Work out the finished part from the listing and answer in its coordinate system (mm). Round coordinates to 2 decimals unless told otherwise and drop trailing zeros. Loops run counter-clockwise (first coordinate to the right, second up) from the corner with the lowest first, then second, coordinate; pieces in that order, holes last. Notation, with made-up numbers: (61.25, 34.25) - (90.25, 34.25) arc R29 cw to (90.25, 57.25) - close; hole circle Ø9 at (-29, 7.25). An arc over 180 degrees is marked (long way). Return JSON: item names as keys, results as strings.
from build123d import *

# Parameters (mm, degrees)
EXTRUDE_1_DEPTH     = 3
SKETCH_2_R          = 1.5
CUT_EXTRUDE_1_DEPTH = 3
SKETCH_3_W          = 11
SKETCH_3_H          = 29.457142857
CUT_EXTRUDE_2_DEPTH = 3
SKETCH_4_W          = 11
SKETCH_4_H          = 29.457142857
CUT_EXTRUDE_3_DEPTH = 3
CUT_EXTRUDE_4_DEPTH = 3


with BuildPart() as part:
    # 草图1 → 凸台-拉伸1 (new body)
    with BuildSketch(Plane.XY):
        Polygon((0, 0), (15, 0), (32.5, -23), (32.5, -38), (-17.5, -38), (-17.5, -23), align=None)
    extrude(amount=EXTRUDE_1_DEPTH)

    # 草图2 → 切除-拉伸1 (cut)
    with BuildSketch(Plane.XY.offset(3)):
        with Locations((7.5, -4)):
            Circle(SKETCH_2_R)
        with Locations((7.5, -17)):
            Circle(SKETCH_2_R)
        with Locations((28.5, -30.5)):
            Circle(SKETCH_2_R)
        with Locations((16.5, -30.5)):
            Circle(SKETCH_2_R)
        with Locations((-1.5, -30.5)):
            Circle(SKETCH_2_R)
        with Locations((-13.5, -30.5)):
            Circle(SKETCH_2_R)
    extrude(amount=-CUT_EXTRUDE_1_DEPTH, mode=Mode.SUBTRACT)

    # 草图3 → 切除-拉伸2 (cut)
    with BuildSketch(Plane.XY.offset(3)):
        with Locations((27, -23.271428571)):
            Rectangle(SKETCH_3_W, SKETCH_3_H)
    extrude(amount=-CUT_EXTRUDE_2_DEPTH, mode=Mode.SUBTRACT)

    # 草图4 → 切除-拉伸3 (cut)
    with BuildSketch(Plane.XY.offset(3)):
        with Locations((-12, -23.271428571)):
            Rectangle(SKETCH_4_W, SKETCH_4_H)
    extrude(amount=-CUT_EXTRUDE_3_DEPTH, mode=Mode.SUBTRACT)

    # 草图5 → 切除-拉伸4 (cut)
    with BuildSketch(Plane.XY.offset(3)):
        Polygon((-6.5, -23), (-6.5, -8.542857143), (0, 0), align=None)
        Polygon((21.5, -23), (21.5, -8.542857143), (15, 0), align=None)
    extrude(amount=-CUT_EXTRUDE_4_DEPTH, mode=Mode.SUBTRACT)


solid = part.part
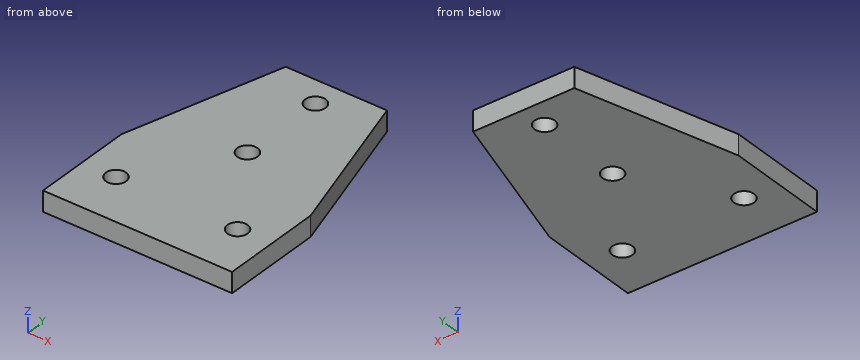
1) Section B-B (x = 7.5) is taken. Give the vertices of the cut face in (y, z).
Verdict:
{"outline": "(-38, 0) - (-18.5, 0) - (-18.5, 3) - (-38, 3) - close; (-15.5, 0) - (-5.5, 0) - (-5.5, 3) - (-15.5, 3) - close; (-2.5, 0) - (0, 0) - (0, 3) - (-2.5, 3) - close"}
2) Find the intervals of material crossed by L1, parallel to Y at x = 7.5, z = 2.25; L2, parallel to Y at x = 8.5, z = 0.35; L3, parallel to X at y = -22.5, z = 2.05, in increasing order.
Verdict:
{"L1": "y = -38 to -18.5, -15.5 to -5.5, -2.5 to 0", "L2": "y = -38 to -18.12, -15.88 to -5.12, -2.88 to 0", "L3": "x = -6.36 to 21.36"}
3) Section C-C (z = 2.05) is taken. Give the vertices of the cut face in (x, y).
Verdict:
{"outline": "(-6.5, -38) - (21.5, -38) - (21.5, -23) - (15, 0) - (0, 0) - (-6.5, -23) - close; hole circle Ø3 at (-1.5, -30.5); hole circle Ø3 at (7.5, -17); hole circle Ø3 at (7.5, -4); hole circle Ø3 at (16.5, -30.5)"}
4) Section A-A (y = -30.5) is taken. Give the vertices of the cut face in (x, z), and give its area (3 significant figures).
Verdict:
{"outline": "(-6.5, 0) - (-3, 0) - (-3, 3) - (-6.5, 3) - close; (0, 0) - (15, 0) - (15, 3) - (0, 3) - close; (18, 0) - (21.5, 0) - (21.5, 3) - (18, 3) - close", "area": "66.0 mm2"}
5) Section D-D (x = -1.5) is taken. Give the vertices of the cut face in (y, z).
Verdict:
{"outline": "(-38, 0) - (-32, 0) - (-32, 3) - (-38, 3) - close; (-29, 0) - (-5.31, 0) - (-5.31, 3) - (-29, 3) - close"}
